Source: CAD feature listing. Evaluate the final solid. Frame: model axes, mm. Face numbers are marked on the shaded views. A direction names the side the tool comes from. Coordinates: 2 decimals unless noted, no trailing zeros. Order: outer loops, then holes, each group sorted by start corner. A loop starts at its lowest first (then second) coordinate and runs counter-clockwise, first axis right, second up. Notation, with made-up numbers: (9, 40.25) -> (34, 40.25) arc R24 cw to (34, 71.25) -> close; hole circle Ø8 at (51.5, 89.5). An arc over 180 degrees is marked (long way). Write each question's results on one line, items separated by ' | '. Start each with the question number.
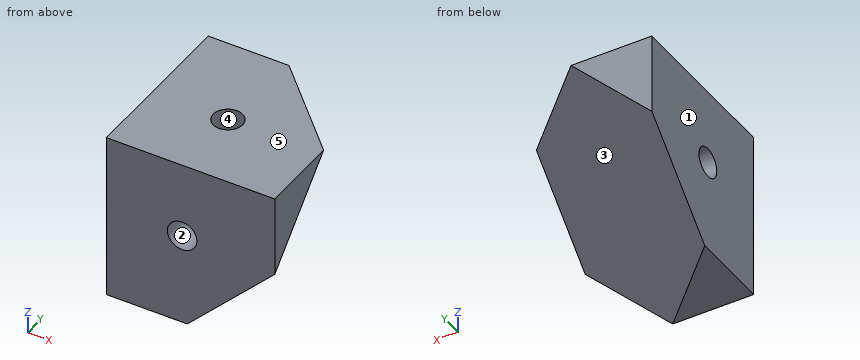
from build123d import *

# Parameters (mm, degrees)
ESQUISSE1_W                  = 20
ESQUISSE1_H                  = 20
BOSS_EXTRU_1_DEPTH           = 20
ESQUISSE2_W                  = 32.659863237
ESQUISSE2_H                  = 28.284271247
ENL_V_MAT_EXTRU_1_DEPTH      = 6
ENL_V_MAT_EXTRU_1_DEPTH_BACK = 12.547005384
ESQUISSE4_R                  = 1.75
ENL_V_MAT_EXTRU_2_DEPTH      = 1
ENL_V_MAT_EXTRU_2_DEPTH_BACK = 8
ESQUISSE5_R                  = 1.75
ENL_V_MAT_EXTRU_3_DEPTH      = 1
ENL_V_MAT_EXTRU_3_DEPTH_BACK = 8
ESQUISSE6_R                  = 1.75
ENL_V_MAT_EXTRU_4_DEPTH      = 1
ENL_V_MAT_EXTRU_4_DEPTH_BACK = 8


with BuildPart() as part:
    # Esquisse1 → Boss.-Extru.1 (new body)
    with BuildSketch(Plane.XY):
        with Locations((10, 10)):
            Rectangle(ESQUISSE1_W, ESQUISSE1_H)
    extrude(amount=BOSS_EXTRU_1_DEPTH)

    # Esquisse2 → Enlèv. mat.-Extru.1 (cut, two sides)
    with BuildSketch(Plane(origin=(6.666666667, 6.666666667, -6.666666667), x_dir=(0.816496581, -0.40824829, 0.40824829), z_dir=(-0.577350269, -0.577350269, 0.577350269))) as enl_v_mat_extru_1_sk:
        with Locations((8.164965809, 14.142135624)):
            Rectangle(ESQUISSE2_W, ESQUISSE2_H)
    extrude(amount=ENL_V_MAT_EXTRU_1_DEPTH, mode=Mode.SUBTRACT)
    extrude(enl_v_mat_extru_1_sk.sketch, amount=-ENL_V_MAT_EXTRU_1_DEPTH_BACK, mode=Mode.SUBTRACT)

    # Esquisse4 → Enlèv. mat.-Extru.2 (cut, two sides)
    with BuildSketch(Plane.XZ) as enl_v_mat_extru_2_sk:
        with Locations((9, 11)):
            Circle(ESQUISSE4_R)
    extrude(amount=ENL_V_MAT_EXTRU_2_DEPTH, mode=Mode.SUBTRACT)
    extrude(enl_v_mat_extru_2_sk.sketch, amount=-ENL_V_MAT_EXTRU_2_DEPTH_BACK, mode=Mode.SUBTRACT)

    # Esquisse5 → Enlèv. mat.-Extru.3 (cut, two sides)
    with BuildSketch(Plane.XY.offset(20)) as enl_v_mat_extru_3_sk:
        with Locations((9, 9)):
            Circle(ESQUISSE5_R)
    extrude(amount=ENL_V_MAT_EXTRU_3_DEPTH, mode=Mode.SUBTRACT)
    extrude(enl_v_mat_extru_3_sk.sketch, amount=-ENL_V_MAT_EXTRU_3_DEPTH_BACK, mode=Mode.SUBTRACT)

    # Esquisse6 → Enlèv. mat.-Extru.4 (cut, two sides)
    with BuildSketch(Plane.ZY) as enl_v_mat_extru_4_sk:
        with Locations((11, 9)):
            Circle(ESQUISSE6_R)
    extrude(amount=ENL_V_MAT_EXTRU_4_DEPTH, mode=Mode.SUBTRACT)
    extrude(enl_v_mat_extru_4_sk.sketch, amount=-ENL_V_MAT_EXTRU_4_DEPTH_BACK, mode=Mode.SUBTRACT)


solid = part.part
(1) Line query: L1, parallel to X at y = 9, z = 18; L2, parallel to X at y = 9, z = 17; L3, parallel to Z at x = 9, y = 2.75. Output: solid intervals per line, ascending.
(2) First-contact query: P1, Ø5.5, axis at x = 9, z = 11, coming from the +Y side; P2, Ø3, axis at x = 9, y = 9, coming from the -Z side; P3, Ø0.8, axis at x = 10, z = 10.5, coming from the -Y side. Flat tips, straight axial feed; report the tip coordinate or a pass-through.
(3) Draft query along X for the marked faces 1, 2 and 3. Return one class per face: released by +X, released by -X, zero draft, split by the parting line, or undercut.
(4) Section C-C on z = 17. Return the cut outline in (x, y).
(5) Reachability of the marked faces 4 and 5 from +Z, -Z, +X, -X, +Y, -Y: full face, straight path, thin tool, end or side. Return the list, or none.
(6) Section B-B on y = 9. Return the cut outline in (x, z).
(7) Section A-A on z = 11. Return the cut outline in (x, y), then the cut area to 3 significant figures.
(8) Section D-D on x = 12. Return the cut outline in (y, z), then the cut area to 3 significant figures.
Results list:
1) L1: x = 0 to 7.25, 10.75 to 18.61 | L2: x = 0 to 7.25, 10.75 to 17.61 | L3: z = 2.14 to 9.25, 12.75 to 20
2) P1: stops at y = 15.5 | P2: stops at z = 6.27 | P3: stops at y = 8
3) face 1: released by -X | face 2: undercut | face 3: released by +X
4) outline: (0, 0) -> (20, 0) -> (20, 6.61) -> (6.61, 20) -> (0, 20) -> close; hole circle Ø3.5 at (9, 9)
5) face 4: +Z | face 5: +Z, +X, -X, +Y, -Y
6) outline: (0, 0) -> (0.61, 0) -> (20, 19.39) -> (20, 20) -> (10.75, 20) -> (10.75, 12) -> (8, 12) -> (8, 9.25) -> (0, 9.25) -> close; (0, 12.75) -> (7.25, 12.75) -> (7.25, 20) -> (0, 20) -> close
7) outline: (0, 0) -> (7.25, 0) -> (7.25, 7.25) -> (0, 7.25) -> close; (0, 10.75) -> (8, 10.75) -> (8, 8) -> (10.75, 8) -> (10.75, 0) -> (20, 0) -> (20, 0.61) -> (0.61, 20) -> (0, 20) -> close | area: 157 mm²
8) outline: (0, 2.39) -> (17.61, 20) -> (0, 20) -> close | area: 155 mm²
